```python
from build123d import *

# Parameters (mm, degrees)
MODEL_R             = 1.5
MODEL_R_2           = 2
EXTRUDE_1_DEPTH     = 2
SKETCH_1_R          = 1.5
CUT_EXTRUDE_1_DEPTH = 2
SKETCH_2_R          = 1.75
CUT_EXTRUDE_2_DEPTH = 10
SKETCH_3_R          = 1.75
CUT_EXTRUDE_3_DEPTH = 10
SKETCH_4_R          = 1.75
CUT_EXTRUDE_4_DEPTH = 10


with BuildPart() as part:
    # Model → 凸台-拉伸1 (new body)
    with BuildSketch(Plane.XY):
        with BuildLine():
            Line((2310.044763103, 1913.686306773), (2310.061692874, 1973.704377759))
            ThreePointArc((2310.061692874, 1973.704377759), (2310.137921285, 1974.087039704), (2310.35478554, 1974.411401894))
            Line((2310.35478554, 1974.411401894), (2352.80617543, 2016.838849342))
            ThreePointArc((2352.80617543, 2016.838849342), (2353.130529599, 2017.055476626), (2353.513082724, 2017.131543129))
            Line((2353.513082724, 2017.131543129), (2359.09903439, 2017.131543129))
            Line((2359.09903439, 2017.131543129), (2413.531484169, 2017.114496472))
            ThreePointArc((2413.531484169, 2017.114496472), (2413.914146114, 2017.038268061), (2414.238508304, 2016.821403806))
            Line((2414.238508304, 2016.821403806), (2456.665838951, 1974.370130782))
            ThreePointArc((2456.665838951, 1974.370130782), (2456.882520181, 1974.045646299), (2456.958532699, 1973.66294141))
            Line((2456.958532699, 1973.66294141), (2456.941602882, 1913.644705177))
            ThreePointArc((2456.941602882, 1913.644705177), (2456.865374471, 1913.262043231), (2456.648510216, 1912.937681042))
            Line((2456.648510216, 1912.937681042), (2435.982160618, 1892.282987197))
            ThreePointArc((2435.982160618, 1892.282987197), (2435.548531394, 1891.634502283), (2435.395975499, 1890.86945739))
            Line((2435.395975499, 1890.86945739), (2435.385853308, 1872.169989535))
            ThreePointArc((2435.385853308, 1872.169989535), (2435.422265409, 1871.702372721), (2435.531117903, 1871.246146395))
            Line((2435.531117903, 1871.246146395), (2456.832006312, 1805.309121837))
            ThreePointArc((2456.832006312, 1805.309121837), (2456.868292251, 1805.15703511), (2456.880427831, 1805.001151277))
            Line((2456.880427831, 1805.001151277), (2456.855314427, 1760.486136893))
            ThreePointArc((2456.855314427, 1760.486136893), (2456.80382295, 1760.169948963), (2456.654989684, 1759.886268089))
            Line((2456.654989684, 1759.886268089), (2442.15029156, 1740.568464651))
            ThreePointArc((2442.15029156, 1740.568464651), (2441.797466901, 1740.274288933), (2441.350345809, 1740.168897647))
            Line((2441.350345809, 1740.168897647), (2325.54447705, 1740.200241027))
            ThreePointArc((2325.54447705, 1740.200241027), (2325.097413073, 1740.305874328), (2324.744747705, 1740.600240991))
            Line((2324.744747705, 1740.600240991), (2310.244646216, 1759.933709642))
            ThreePointArc((2310.244646216, 1759.933709642), (2310.095962918, 1760.217481876), (2310.044646216, 1760.533709642))
            Line((2310.044646216, 1760.533709642), (2310.044646216, 1805.042570403))
            ThreePointArc((2310.044646216, 1805.042570403), (2310.056869737, 1805.198447365), (2310.093241471, 1805.350513596))
            Line((2310.093241471, 1805.350513596), (2331.434636288, 1871.285740281))
            ThreePointArc((2331.434636288, 1871.285740281), (2331.543751489, 1871.741938976), (2331.580422052, 1872.209569862))
            Line((2331.580422052, 1872.209569862), (2331.580422052, 1890.907725019))
            ThreePointArc((2331.580422052, 1890.907725019), (2331.428181117, 1891.673091884), (2330.994635614, 1892.321938582))
            Line((2330.994635614, 1892.321938582), (2310.337656282, 1912.978917914))
            ThreePointArc((2310.337656282, 1912.978917914), (2310.120829567, 1913.303471569), (2310.044763103, 1913.686306773))
        make_face()
        with Locations((2359.09903439, 2008.131543129)):
            Circle(MODEL_R, mode=Mode.SUBTRACT)
        with Locations((2407.945697715, 2008.131543129)):
            Circle(MODEL_R, mode=Mode.SUBTRACT)
        with Locations((2348.501647878, 1978.674541468)):
            Circle(MODEL_R_2, mode=Mode.SUBTRACT)
        with Locations((2348.501647878, 1908.674541468)):
            Circle(MODEL_R_2, mode=Mode.SUBTRACT)
        with Locations((2418.543084227, 1978.674541468)):
            Circle(MODEL_R_2, mode=Mode.SUBTRACT)
        with Locations((2418.543084227, 1908.674541468)):
            Circle(MODEL_R_2, mode=Mode.SUBTRACT)
        with Locations((2412.471188929, 1828.036421631)):
            Circle(MODEL_R, mode=Mode.SUBTRACT)
        with Locations((2317.78863196, 1972.045859296)):
            Circle(MODEL_R_2, mode=Mode.SUBTRACT)
        with Locations((2449.230659179, 1972.008782408)):
            Circle(MODEL_R_2, mode=Mode.SUBTRACT)
        with Locations((2354.471188929, 1828.036421631)):
            Circle(MODEL_R, mode=Mode.SUBTRACT)
        with Locations((2354.471188929, 1779.036421631)):
            Circle(MODEL_R, mode=Mode.SUBTRACT)
        with Locations((2412.471188929, 1779.036421631)):
            Circle(MODEL_R, mode=Mode.SUBTRACT)
        with Locations((2327.144646216, 1757.400376309)):
            Circle(MODEL_R_2, mode=Mode.SUBTRACT)
        with Locations((2439.750176643, 1757.400376309)):
            Circle(MODEL_R_2, mode=Mode.SUBTRACT)
        with Locations((2317.772636576, 1915.340300528)):
            Circle(MODEL_R_2, mode=Mode.SUBTRACT)
        with Locations((2449.207368346, 1915.286332047)):
            Circle(MODEL_R_2, mode=Mode.SUBTRACT)
        with Locations((2348.478614662, 1857.106083087)):
            Circle(MODEL_R, mode=Mode.SUBTRACT)
        with Locations((2418.478612099, 1857.087137272)):
            Circle(MODEL_R, mode=Mode.SUBTRACT)
        with Locations((2362.47861415, 1857.102293924)):
            Circle(MODEL_R, mode=Mode.SUBTRACT)
        with Locations((2404.478612663, 1857.091119611)):
            Circle(MODEL_R, mode=Mode.SUBTRACT)
        with BuildLine():
            Line((2376.022366052, 2009.631543129), (2391.022366052, 2009.631543129))
            ThreePointArc((2391.022366052, 2009.631543129), (2392.522366052, 2008.131543129), (2391.022366052, 2006.631543129))
            Line((2391.022366052, 2006.631543129), (2376.022366052, 2006.631543129))
            ThreePointArc((2376.022366052, 2006.631543129), (2374.522366052, 2008.131543129), (2376.022366052, 2009.631543129))
        make_face(mode=Mode.SUBTRACT)
        with BuildLine():
            Line((2348.450119256, 1751.694041878), (2418.450116692, 1751.675096064))
            ThreePointArc((2418.450116692, 1751.675096064), (2419.949710601, 1750.174690192), (2418.450116692, 1748.675096064))
            Line((2418.450116692, 1748.675096064), (2348.450119256, 1748.694041878))
            ThreePointArc((2348.450119256, 1748.694041878), (2346.950525348, 1750.19444775), (2348.450119256, 1751.694041878))
        make_face(mode=Mode.SUBTRACT)
    extrude(amount=EXTRUDE_1_DEPTH)

    # 草图1 → 切除-拉伸1 (cut)
    with BuildSketch(Plane(origin=(0, 0, 0), x_dir=(-1, 0, 0), z_dir=(0, 0, -1))):
        with Locations((-2404.471188929, 1842.036421631)):
            Circle(SKETCH_1_R)
        with Locations((-2362.471188929, 1842.036421631)):
            Circle(SKETCH_1_R)
        with Locations((-2362.471188929, 1779.036421631)):
            Circle(SKETCH_1_R)
        with Locations((-2404.471188929, 1779.036421631)):
            Circle(SKETCH_1_R)
    extrude(amount=-CUT_EXTRUDE_1_DEPTH, mode=Mode.SUBTRACT)

    # 草图2 → 切除-拉伸2 (cut)
    with BuildSketch(Plane(origin=(0, 0, 0), x_dir=(-1, 0, 0), z_dir=(0, 0, -1))):
        with Locations((-2428.510112786, 1880.172373647)):
            Circle(SKETCH_2_R)
        with Locations((-2338.510112786, 1880.172373647)):
            Circle(SKETCH_2_R)
        with Locations((-2428.510112786, 1760.172373647)):
            Circle(SKETCH_2_R)
        with Locations((-2338.510112786, 1760.172373647)):
            Circle(SKETCH_2_R)
    extrude(amount=-CUT_EXTRUDE_2_DEPTH, mode=Mode.SUBTRACT)

    # 草图3 → 切除-拉伸3 (cut)
    with BuildSketch(Plane(origin=(0, 0, 0), x_dir=(-1, 0, 0), z_dir=(0, 0, -1))):
        with Locations((-2444.956091075, 1965.008782408)):
            Circle(SKETCH_3_R)
        with Locations((-2424.956091075, 1965.008782408)):
            Circle(SKETCH_3_R)
        with Locations((-2444.944525882, 1924.008782408)):
            Circle(SKETCH_3_R)
        with Locations((-2424.944525882, 1924.008782408)):
            Circle(SKETCH_3_R)
        with Locations((-2403.950117974, 2005.117496488)):
            Circle(SKETCH_3_R)
        with Locations((-2362.950119985, 2005.130336493)):
            Circle(SKETCH_3_R)
        with Locations((-2403.950117974, 1985.117496488)):
            Circle(SKETCH_3_R)
        with Locations((-2362.950119985, 1985.130336493)):
            Circle(SKETCH_3_R)
        with Locations((-2342.059240516, 1965.008782408)):
            Circle(SKETCH_3_R)
        with Locations((-2322.059240516, 1965.008782408)):
            Circle(SKETCH_3_R)
        with Locations((-2342.047675323, 1924.008784039)):
            Circle(SKETCH_3_R)
        with Locations((-2322.047675323, 1924.008784039)):
            Circle(SKETCH_3_R)
        with Locations((-2442.856091075, 1947.008782408)):
            Circle(SKETCH_3_R)
        with Locations((-2427.056091075, 1947.008782408)):
            Circle(SKETCH_3_R)
        with Locations((-2339.959240516, 1947.008782408)):
            Circle(SKETCH_3_R)
        with Locations((-2324.159240516, 1947.008782408)):
            Circle(SKETCH_3_R)
        with Locations((-2383.450117974, 2003.017496488)):
            Circle(SKETCH_3_R)
        with Locations((-2383.450117974, 1987.217496488)):
            Circle(SKETCH_3_R)
    extrude(amount=-CUT_EXTRUDE_3_DEPTH, mode=Mode.SUBTRACT)

    # 草图4 → 切除-拉伸4 (cut)
    with BuildSketch(Plane(origin=(0, 0, 0), x_dir=(-1, 0, 0), z_dir=(0, 0, -1))):
        with Locations((-2398.450117974, 1977.180510087)):
            Circle(SKETCH_4_R)
        with Locations((-2398.450117974, 1877.180510087)):
            Circle(SKETCH_4_R)
        with Locations((-2398.450117974, 1777.180510087)):
            Circle(SKETCH_4_R)
        with Locations((-2368.450117974, 1977.188629722)):
            Circle(SKETCH_4_R)
        with Locations((-2368.450117974, 1877.188629722)):
            Circle(SKETCH_4_R)
        with Locations((-2368.450117974, 1777.188629722)):
            Circle(SKETCH_4_R)
    extrude(amount=-CUT_EXTRUDE_4_DEPTH, mode=Mode.SUBTRACT)


solid = part.part
```
Here's how the part is built. I have some questions about the finished solid (model axes, mm). A direction names the side the tool comes from. Give positions to 0.01 mm unless a question says otherwise; leave off trailing zeros. Write each loop counter-clockwise with the first axis right and the second up, starting at its lowest first coordinate (ties: lowest second). Pieces come first, ordered by that corner, then holes. Notation, with made-up numbers: (-4.5, 1) -> (3.5, 1) arc R34 ccw to (3.5, 38) -> close; hole circle Ø11 at (53.25, 68.25). An arc over 180 degrees is marked (long way). Use one line per item in the form item = value.
1) We'd pull the mould along Y, two halves only. Please class faces 4 (the face through (2385, 1881, 2)), 5 (the face through (2320.615, 1837.857, 0.986)), 6 (the face through (2331.283, 1995.328, 0.986)): +Y half, -Y half, draft (parallel to the pull), parting line (faces both ways), or undercut.
Verdict:
face_4 = draft
face_5 = undercut
face_6 = +Y half
2) On a 3-axis mill with a long thin cutter (end or side, diameter ignored), from which of +Z, -Z, +X, -X, +Y, -Y can I reach the whole of each face in a straight line? I mean faces 1 (the face through (2446.032, 1838.739, 0.986)), 2 (the face through (2320.811, 1902.506, 0.986)), 3 (the face through (2385, 1881, 0)). Say none if no direction works.
Verdict:
face_1 = +Z, -Z, +X
face_2 = +Z, -Z, -X
face_3 = -Z, +X, -X, +Y, -Y
3) I'm going to push flat-ended pins straight in: pin 1 (2.5 mm diameter, centred on x = 2354.47, y = 1828.04, fed in from -Z); pin 2 (0.6 mm diameter, centred on x = 2397, z = 1.5, fed in from +Y). Where does each tip first touch, or does it pass through?
Verdict:
pin_1 = through
pin_2 = 2017.12
4) Suppose I cut it at A-A (z = 0.45). Give the number of separate pieces and of enclosed holes in the cut face, and give its area (3 significant figures).
Verdict:
separate_pieces = 1
enclosed_holes = 54
area = 35,000 mm2
5) If I drill on L1, parallel to Y at x = 2368, z = 0.3; L2, parallel to Y at x = 2378.5, z = 0.9; L3, parallel to Y at x = 2426.5, z = 1.4, over which ranges is the centre line in solid material (lowest first)? Write a range as [from, to].
Verdict:
L1 = [1740.19, 1748.69], [1751.69, 1775.5], [1778.88, 1875.5], [1878.88, 1975.5], [1978.88, 2017.13]
L2 = [1740.19, 1748.69], [1751.69, 2006.63], [2009.63, 2017.13]
L3 = [1740.17, 1923.21], [1924.81, 1945.35], [1948.67, 1964.18], [1965.83, 2004.55]
6) Suppose I cut it at B-B (y = 1897.5). Please give me the cut outline in (x, z), and give its area (3 significant figures).
Verdict:
outline = (2325.82, 0) -> (2441.2, 0) -> (2441.2, 2) -> (2325.82, 2) -> close
area = 231 mm2
